from build123d import *

# Parameters (mm, degrees)
F1_DEPTH = 2
F0_W     = 1
F0_H     = 10
F2_DEPTH = 7
F3_R     = 1.5
F4_DEPTH = 2
F5_DEPTH = 25


with BuildPart() as f1:
    # F0 (on Front) → F1 (new body)
    with BuildSketch(Plane.XZ):
        Polygon((-95, -50), (95, -50), (95, -40), (94, -40), (94, -30), (95, -30), (95, 30), (94, 30), (94, 40), (95, 40), (95, 50), (-95, 50), align=None)
    extrude(amount=F1_DEPTH)



with BuildPart() as f2:
    # F0 (on Front) → F2 (new body)
    with BuildSketch(Plane.XZ):
        with Locations((94.5, 35)):
            Rectangle(F0_W, F0_H)
    extrude(amount=F2_DEPTH)


with BuildPart() as f2b:
    # F0 (on Front) → F2, piece 2 (new body)
    with BuildSketch(Plane.XZ):
        with Locations((94.5, -35)):
            Rectangle(F0_W, F0_H)
    extrude(amount=F2_DEPTH)


with BuildPart() as f1_1:
    add(f1.part)

    add(f2.part)  # F4 merges F2

    add(f2b.part)  # F4 merges F2b
    # F3 (on face) → F4 (join)
    with BuildSketch(Plane.YZ.offset(95)):
        with BuildLine():
            Line((0, -30), (-7, -30))
            ThreePointArc((-7, -30), (-12, -35), (-7, -40))
            Line((-7, -40), (0, -40))
            Line((0, -40), (0, -30))
        make_face()
        with Locations((-7, -35)):
            Circle(F3_R, mode=Mode.SUBTRACT)
        with BuildLine():
            Line((0, 40), (-7, 40))
            Line((-7, 40), (-7, 36.5))
            ThreePointArc((-7, 36.5), (-5.9393398282, 36.0606601718), (-5.5, 35))
            ThreePointArc((-5.5, 35), (-5.9393398282, 33.9393398282), (-7, 33.5))
            Line((-7, 33.5), (-7, 30))
            Line((-7, 30), (0, 30))
            Line((0, 30), (0, 40))
        make_face()
        with Locations((-7, -35)):
            Circle(F3_R)
        with BuildLine():
            Line((-7, 36.5), (-7, 40))
            ThreePointArc((-7, 40), (-12, 35), (-7, 30))
            Line((-7, 30), (-7, 33.5))
            ThreePointArc((-7, 33.5), (-8.5, 35), (-7, 36.5))
        make_face()
        with BuildLine():
            ThreePointArc((-5.5, 35), (-5.9393398282, 36.0606601718), (-7, 36.5))
            Line((-7, 36.5), (-7, 33.5))
            ThreePointArc((-7, 33.5), (-5.9393398282, 33.9393398282), (-5.5, 35))
        make_face()
        with BuildLine():
            Line((-7, 33.5), (-7, 36.5))
            ThreePointArc((-7, 36.5), (-8.5, 35), (-7, 33.5))
        make_face()
    extrude(amount=-F4_DEPTH)

    # F3 (on face) → F5 (cut)
    with BuildSketch(Plane.YZ.offset(95)):
        with Locations((-7, -35)):
            Circle(F3_R)
        with BuildLine():
            Line((-7, 33.5), (-7, 36.5))
            ThreePointArc((-7, 36.5), (-8.5, 35), (-7, 33.5))
        make_face()
        with BuildLine():
            ThreePointArc((-5.5, 35), (-5.9393398282, 36.0606601718), (-7, 36.5))
            Line((-7, 36.5), (-7, 33.5))
            ThreePointArc((-7, 33.5), (-5.9393398282, 33.9393398282), (-5.5, 35))
        make_face()
    extrude(amount=-F5_DEPTH, mode=Mode.SUBTRACT)


solid = f1_1.part
Model file for the job. Use its own axes, mm. A direction names the side the tool comes from. Give positions to 0.01 mm unless a question says otherwise; leave off trailing zeros. Order: outer loops, then holes, each group sorted by start corner. A loop starts at its lowest first (then second) coordinate and runs counter-clockwise, first axis right, second up. Notation, with made-up numbers: (-22.75, -0.75) -> (-3.75, -0.75) arc R26 cw to (-3.75, 14.25) -> close; hole circle Ø10 at (43.25, 59). An arc over 180 degrees is marked (long way). Use CSV: the item, a comma, the result in double quotes.
1. Band-saw the part on B-B, the plane z = -43. Give the cut face in (x, y), then the cut area to 3 significant figures.
Outcome:
outline,"(-95, -2) -> (95, -2) -> (95, 0) -> (-95, 0) -> close"
area,"380 mm²"
2. Band-saw the part on A-A, the plane x = 9.5. Give the cut face in (y, z), then the cut area to 3 significant figures.
Outcome:
outline,"(-2, -50) -> (0, -50) -> (0, 50) -> (-2, 50) -> close"
area,"200 mm²"
3. Drop flat-ended pins along their axis: pin 1 (4 mm diameter, centred on y = -9.5, z = -37.5, fed in from -X); pin 2 (0.6 mm diameter, centred on x = 93.5, y = -4.5, fed in from +Z); pin 3 (1 mm diameter, centred on x = 41, z = 11, fed in from -Y); pin 4 (12 mm diameter, centred on x = 9.5, z = 37, fed in from +Y). Give the stop position or say it passes through.
Outcome:
pin 1,"x = 93"
pin 2,"z = 40"
pin 3,"y = -2"
pin 4,"y = 0"
4. Drill centre lines: line 1 along Z through (x, y) = (94.35, -7); line 2 along Y through (x, z) = (-10, 13). Where is each one in solid material? Low to high. Write a range as from..to.
Outcome:
line 1,"-40..-36.5, -33.5..-30, 30..33.5, 36.5..40"
line 2,"-2..0"
5. Mould opens along Z. For faces 1 (the cylindrical face through (94, -12, -35)), 2 (the flat face through (95, -1, -1)), 3 (the cylindrical face through (94, -12, 35)) say: +Z half, -Z half, draft (parallel to the pull), parting line (faces both ways), or undercut.
Outcome:
face 1,"undercut"
face 2,"draft"
face 3,"undercut"
6. 3-axis set-ups, long thin cutter, end or side, ignore diameter. For faces 4 (the flat face through (93, -5, -35)), 5 (the flat face through (1, 0, -1)): which of +Z, -Z, +X, -X, +Y, -Y reach the whole face in a straight line?
Outcome:
face 4,"+Z, -Z, -X, -Y"
face 5,"+Z, -Z, +X, -X, +Y"
